```python
from build123d import *

# Parameters (mm, degrees)
SKETCH_R      = 2.5
PAD_DEPTH     = 0.6
SKETCH002_R   = 8
SKETCH002_R_2 = 2.5
PAD001_DEPTH  = 1


with BuildPart() as part:
    # Sketch → Pad (new body)
    with BuildSketch(Plane.XY):
        with BuildLine():
            ThreePointArc((-2.5, 3.122499), (-3.518971, 1.901799), (-3.981855, 0.380567))
            Line((-5.478695, -0.483634), (-3.981855, 0.380567))
            ThreePointArc((-5.478695, -0.483634), (-4.659167, -2.922699), (-2.81991, -4.722087))
            Line((-1.232265, -3.80546), (-2.81991, -4.722087))
            ThreePointArc((-1.232265, -3.80546), (0.117848, -3.998264), (1.454262, -3.726275))
            Line((2.992718, -4.614503), (1.454262, -3.726275))
            ThreePointArc((2.992718, -4.614503), (4.763149, -2.749985), (5.492638, -0.284484))
            Line((3.954108, 0.604177), (5.492638, -0.284484))
            ThreePointArc((3.954108, 0.604177), (3.46401, 2.000159), (2.5, 3.122499))
            Line((2.5, 3.122499), (2.5, 4.898979))
            ThreePointArc((2.5, 4.898979), (0, 5.5), (-2.5, 4.898979))
            Line((-2.5, 3.122499), (-2.5, 4.898979))
        make_face()
        Circle(SKETCH_R, mode=Mode.SUBTRACT)
    extrude(amount=PAD_DEPTH)

    # Sketch002 (on Face15 of Pad) → Pad001 (join)
    with BuildSketch(Plane.XY.offset(0.6)):
        Circle(SKETCH002_R)
        Circle(SKETCH002_R_2, mode=Mode.SUBTRACT)
    extrude(amount=PAD001_DEPTH)


solid = part.part
```
Work out the finished part from the listing and answer in its coordinate system (mm). A direction names the side the tool comes from. Coordinates: 2 decimals unless noted, no trailing zeros. Loops run counter-clockwise (first coordinate to the right, second up) from the corner with the lowest first, then second, coordinate; pieces in that order, holes last.
1) Consider probe 1 along X at (y, z) = (-0.5, 1.25); probe 2 along Z at (x, y) = (4.75, -6); probe 3 along X at (y, z) = (2, 1.1). Determine where each line is inside the solid, lowest interval first.
Results:
probe 1: x = -7.98 to -2.45, 2.45 to 7.98
probe 2: z = 0.6 to 1.6
probe 3: x = -7.75 to -1.5, 1.5 to 7.75
2) Section A-A (x = 0) is taken. Give the vertices of the cut face in (y, z).
Results:
outline: (-8, 0.6) - (-4, 0.6) - (-4, 0) - (-2.5, 0) - (-2.5, 1.6) - (-8, 1.6) - close; (2.5, 0) - (5.5, 0) - (5.5, 0.6) - (8, 0.6) - (8, 1.6) - (2.5, 1.6) - close
3) A flat-ended cylindrical pin translates along its axis: pin 1 (0.7 mm diameter, centred on y = 4.5, z = 0.5, fed in from -X). Find the tip coordinate at first contact, or state that the pin passes through.
Results:
pin 1: stops at x = -6.83
4) For a pull along Y with two mould halves and no side action, classify faces 5 (the flat face through (-2.015, -4.257, 0.296)), 6 (the flat face through (4.713, 0.166, 0.296)), 7 (the cylindrical face through (-0.54, -2.44, 0.79)) as +Y half, -Y half, draft (parallel to the pull), parting line (faces both ways), or undercut.
Results:
face 5: -Y half
face 6: +Y half
face 7: undercut
5) For faces 1 (the flat face through (2.234, -4.177, 0.296)), 2 (the flat face through (-4, 2, 0.6)), 3 (the cylindrical face through (-4.68, -2.89, 0.3)), 4 (the flat face through (-4.741, -0.058, 0.296)), determine the directions among +Z, -Z, +X, -X, +Y, -Y from which every point of the face is accessible in a straight line to the end or side of a thin tool.
Results:
face 1: -Z, -Y
face 2: -Z
face 3: -Z, -X, -Y
face 4: -Z, -X, +Y
6) Section C-C (y = -2) is taken. Give the vertices of the cut face in (x, z).
Results:
outline: (-7.75, 0.6) - (-5.12, 0.6) - (-5.12, 0) - (-1.5, 0) - (-1.5, 1.6) - (-7.75, 1.6) - close; (1.5, 0) - (5.12, 0) - (5.12, 0.6) - (7.75, 0.6) - (7.75, 1.6) - (1.5, 1.6) - close
7) Section B-B (z = 0.2) is taken. Give the vertices of the cut face in (x, y), plus the area to 3 significant figures.
Results:
outline: (-5.48, -0.48) arc R5.5 ccw to (-2.82, -4.72) - (-1.23, -3.81) arc R4 ccw to (1.45, -3.73) - (2.99, -4.61) arc R5.5 ccw to (5.49, -0.28) - (3.95, 0.6) arc R4 ccw to (2.5, 3.12) - (2.5, 4.9) arc R5.5 ccw to (-2.5, 4.9) - (-2.5, 3.12) arc R4 ccw to (-3.98, 0.38) - close; hole circle Ø5 at (0, 0)
area: 54.4 mm2
8) Section D-D (y = 3.5) is taken. Give the vertices of the cut face in (x, z), plus the area to 3 significant figures.
Results:
outline: (-7.19, 0.6) - (-2.5, 0.6) - (-2.5, 0) - (2.5, 0) - (2.5, 0.6) - (7.19, 0.6) - (7.19, 1.6) - (-7.19, 1.6) - close
area: 17.4 mm2
